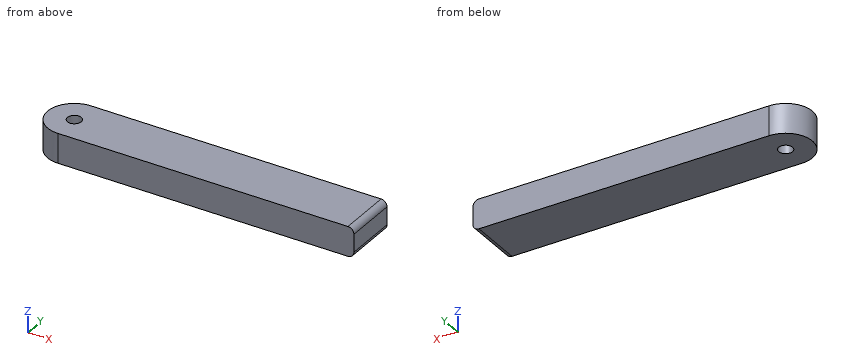
from build123d import *

# Parameters (mm, degrees)
ESQUISSE1_R        = 2.35
BOSS_EXTRU_1_DEPTH = 10
CONG_1_R           = 2


with BuildPart() as part:
    # Esquisse1 → Boss.-Extru.1 (new body)
    with BuildSketch(Plane.XY):
        with BuildLine():
            Line((0, 9), (100, 9))
            Line((100, 9), (100, -9))
            Line((100, -9), (0, -9))
            ThreePointArc((0, -9), (-9, 0), (0, 9))
        make_face()
        Circle(ESQUISSE1_R, mode=Mode.SUBTRACT)
    extrude(amount=BOSS_EXTRU_1_DEPTH)

    # Congé1
    cong_1_edges = [part.edges().sort_by_distance(p)[0] for p in [
        (100, 0, 10),
        (100, 0, 0),
    ]]
    fillet(cong_1_edges, radius=CONG_1_R)


solid = part.part
Build history of the part. All positions in model axes, mm. Give positions to 0.01 mm unless a question says otherwise; leave off trailing zeros. Order: outer loops, then holes, each group sorted by start corner. A loop starts at its lowest first (then second) coordinate and runs counter-clockwise, first axis right, second up. Notation, with made-up numbers: M -24.75,36 L 21.25,36 A31 ccw 21.25,66 Z; hole C 25.5,59.25 d5. An arc over 180 degrees is marked long. Put each result on its own line as item: value.
Item 1: Wall check: probe 1 along X at (y, z) = (-1.75, 5.75); probe 2 along X at (y, z) = (7.25, 5); probe 3 along X at (y, z) = (-7, 8.5). Give the ranges that are in metal, low to high.
Results are:
probe 1: -8.83 to -1.57, 1.57 to 100
probe 2: -5.33 to 100
probe 3: -5.66 to 99.94
Item 2: Drop a flat-ended pin along its axis: pin 1 Ø2 at (y, z) = (-2.5, 4.5) entering from -X. Give the stop position or say it passes through.
Results are:
pin 1: x = -8.87
Item 3: Cut at C-C on y = -7.75. Write the cut outline in (x, z), then the cut area to 3 significant figures.
Results are:
outline: M -4.58,0 L 98,0 A2 ccw 100,2 L 100,8 A2 ccw 98,10 L -4.58,10 Z
area: 1,040 mm2
Item 4: Cut at D-D on z = 9. Write the cut outline in (x, y).
Results are:
outline: M 0,-9 L 99.73,-9 L 99.73,9 L 0,9 A9 ccw Z; hole C 0,0 d4.7
Item 5: Cut at A-A on y = 0. Write the cut outline in (x, z).
Results are:
outline: M -9,0 L -2.35,0 L -2.35,10 L -9,10 Z; M 2.35,0 L 98,0 A2 ccw 100,2 L 100,8 A2 ccw 98,10 L 2.35,10 Z
Item 6: Cut at B-B on z = 4.5. Write the cut outline in (x, y).
Results are:
outline: M 0,-9 L 100,-9 L 100,9 L 0,9 A9 ccw Z; hole C 0,0 d4.7
